Verification items for the finished model (mm, model axes). Coordinates: 2 decimals unless noted, no trailing zeros. Loops run counter-clockwise (first coordinate to the right, second up) from the corner with the lowest first, then second, coordinate; pieces in that order, holes last. Notation, with made-up numbers: (-38, -15.75) -> (8, -15.75) arc R13 cw to (8, 2.25) -> close; hole circle Ø10 at (71.5, 49.5). An arc over 180 degrees is marked (long way). Use CSV: the item, a comma, the result in double quotes. Start each with the question number.
```python
from build123d import *

# Parameters (mm, degrees)
CROQUIS1_R                 = 4.5
CROQUIS1_R_2               = 4
SALIENTE_EXTRUIR1_DEPTH    = 80
CROQUIS2_R                 = 1.5
CORTAR_EXTRUIR1_DEPTH      = 5.5
CORTAR_EXTRUIR1_DEPTH_BACK = 5.5


with BuildPart() as part:
    # Croquis1 → Saliente-Extruir1 (new body)
    with BuildSketch(Plane(origin=(0, 0, 0), x_dir=(1, 0, 0), z_dir=(0, 1, 0))):
        Circle(CROQUIS1_R)
        Circle(CROQUIS1_R_2, mode=Mode.SUBTRACT)
    extrude(amount=SALIENTE_EXTRUIR1_DEPTH)

    # Croquis2 → Cortar-Extruir1 (cut, two sides)
    with BuildSketch(Plane(origin=(0, 0, 0), x_dir=(0, 0, -1), z_dir=(1, 0, 0))) as cortar_extruir1_sk:
        with Locations((0, 75)):
            Circle(CROQUIS2_R)
        with Locations((0, 5)):
            Circle(CROQUIS2_R)
    extrude(amount=CORTAR_EXTRUIR1_DEPTH, mode=Mode.SUBTRACT)
    extrude(cortar_extruir1_sk.sketch, amount=-CORTAR_EXTRUIR1_DEPTH_BACK, mode=Mode.SUBTRACT)


solid = part.part
```
1. Depth check by flat-ended pin: pin 1 (1.5 mm diameter, centred on y = 58.5, z = -1, fed in from -X); pin 2 (1.8 mm diameter, centred on y = 75, z = 0, fed in from +X); pin 3 (2 mm diameter, centred on y = 60.5, z = -2.5, fed in from -X). Enter the tip coordinate at first touch or a pass-through.
2. Cross-section at A-A, the plane z = 0. Record the boundary of the cut face in (x, y), plus the area to 3 significant figures.
3. Cross-section at C-C, the plane y = 5. Record the boundary of the cut face in (x, z).
4. Scan lines: line 1 (Y direction, x = -4.1, z = 0); line 2 (X direction, y = 57, z = 0.25); line 3 (Z direction, x = 0, y = 18.5). Record each from-to range of solid material in increasing order.
5. Cross-section at B-B, the plane x = 0. Record the boundary of the cut face in (y, z).
6. Cross-section at D-D, the plane y = 19. Record the boundary of the cut face in (x, z), plus the area to 3 significant figures.
7. Release check for a two-part mould opening along Z. For faces 1 (the cylindrical face through (4.16, 39.44, 1.72)), 2 (the cylindrical face through (4.1, 5.45, -1.43)), 3 (the flat face through (-3, 0, 3)) record: released by +Z, released by -Z, zero draft, split by the parting line, or undercut.
Solution:
1,pin 1,"stops at x = -4.49"
1,pin 2,"passes through"
1,pin 3,"stops at x = -4.24"
2,outline,"(-4.5, 0) -> (-4, 0) -> (-4, 3.5) -> (-4.5, 3.5) -> close; (-4.5, 6.5) -> (-4, 6.5) -> (-4, 73.5) -> (-4.5, 73.5) -> close; (-4.5, 76.5) -> (-4, 76.5) -> (-4, 80) -> (-4.5, 80) -> close; (4, 0) -> (4.5, 0) -> (4.5, 3.5) -> (4, 3.5) -> close; (4, 6.5) -> (4.5, 6.5) -> (4.5, 73.5) -> (4, 73.5) -> close; (4, 76.5) -> (4.5, 76.5) -> (4.5, 80) -> (4, 80) -> close"
2,area,"74.0 mm2"
3,outline,"(-4.24, -1.5) arc R4.5 ccw to (4.24, -1.5) -> (3.71, -1.5) arc R4 cw to (-3.71, -1.5) -> close; (-4.24, 1.5) -> (-3.71, 1.5) arc R4 cw to (3.71, 1.5) -> (4.24, 1.5) arc R4.5 ccw to start"
4,line 1,"y = 0 to 3.5, 6.5 to 73.5, 76.5 to 80"
4,line 2,"x = -4.49 to -3.99, 3.99 to 4.49"
4,line 3,"z = -4.5 to -4, 4 to 4.5"
5,outline,"(0, -4.5) -> (80, -4.5) -> (80, -4) -> (0, -4) -> close; (0, 4) -> (80, 4) -> (80, 4.5) -> (0, 4.5) -> close"
6,outline,"circle Ø9 at (0, 0); hole circle Ø8 at (0, 0)"
6,area,"13.4 mm2"
7,face 1,"split by the parting line"
7,face 2,"undercut"
7,face 3,"zero draft"
